```python
from build123d import *

# Parameters (mm, degrees)
F1_DEPTH = 33.02
F2_R     = 5.08
F4_T     = -2.032
F3_R     = 2.794
F5_DEPTH = 2.032


with BuildPart() as f1:
    # F0 (on Top) → F1 (new body)
    with BuildSketch(Plane.XY):
        Polygon((-40.064697, 25.4), (-25.4, 0), (-25.4, 25.4), align=None)
        Polygon((-40.064697, 25.4), (-25.4, 25.4), (-25.4, 50.8), align=None)
        Polygon((-25.4, 0), (0, 0), (0, 50.8), (-25.4, 50.8), (-25.4, 25.4), align=None)
    extrude(amount=F1_DEPTH)

    # F2
    f2_edges = [f1.edges().sort_by_distance(p)[0] for p in [
        (-40.064697, 25.4, 16.51),
        (-25.4, 50.8, 16.51),
        (-25.4, 0, 16.51),
    ]]
    fillet(f2_edges, radius=F2_R)

    # F4
    f4_openings = [f1.faces().sort_by_distance(p)[0] for p in [
        (-16.606713, 25.4, 33.02),
    ]]
    offset(amount=F4_T, openings=f4_openings)

    # F3 (on face) → F5 (cut)
    with BuildSketch(Plane(origin=(0, 0, 0), x_dir=(1, 0, 0), z_dir=(0, 0, -1))):
        with Locations((-11.23353, -25.4)):
            Circle(F3_R)
        with Locations((-11.23353, -38.1)):
            Circle(F3_R)
    extrude(amount=-F5_DEPTH, mode=Mode.SUBTRACT)


solid = f1.part
```
Build history of the part. All positions in model axes, mm. A direction names the side the tool comes from. Coordinates: 2 decimals unless noted, no trailing zeros. Order: outer loops, then holes, each group sorted by start corner. A loop starts at its lowest first (then second) coordinate and runs counter-clockwise, first axis right, second up.
Item 1: Tool access for faces 5 (the cylindrical face through (-11.6, 35.33, 1)), 6 (the flat face through (-12, 2.032, 17)): list every direction of +Z, -Z, +X, -X, +Y, -Y with a clear straight run to the whole face (end or side of a thin tool).
Filled in:
face 5: +Z, -Z
face 6: +Z
Item 2: Saw through at C-C on x = -13. List the corners of the cut face in (y, z), then the cut area to 3 significant figures.
Filled in:
outline: (0, 0) - (23.24, 0) - (23.24, 2.03) - (2.03, 2.03) - (2.03, 33.02) - (0, 33.02) - close; (27.56, 0) - (35.94, 0) - (35.94, 2.03) - (27.56, 2.03) - close; (40.26, 0) - (50.8, 0) - (50.8, 33.02) - (48.77, 33.02) - (48.77, 2.03) - (40.26, 2.03) - close
area: 212 mm2
Item 3: Saw through at A-A on y = 24.5. List the corners of the cut face in (x, z), then the cut area to 3 significant figures.
Filled in:
outline: (-39.2, 0) - (-13.88, 0) - (-13.88, 2.03) - (-37.11, 2.03) - (-37.11, 33.02) - (-39.2, 33.02) - close; (-8.59, 0) - (0, 0) - (0, 33.02) - (-2.03, 33.02) - (-2.03, 2.03) - (-8.59, 2.03) - close
area: 197 mm2
Item 4: Saw through at D-D on x = -4. List the corners of the cut face in (y, z), then the cut area to 3 significant figures.
Filled in:
outline: (0, 0) - (50.8, 0) - (50.8, 33.02) - (48.77, 33.02) - (48.77, 2.03) - (2.03, 2.03) - (2.03, 33.02) - (0, 33.02) - close
area: 229 mm2
Item 5: Drill centre lines: L1, parallel to Y at x = -6.5, z = 3; L2, parallel to X at y = 25.4, z = 0.4; L3, parallel to Z at x = -5, y = 9. Where is each one in solid material? Low to high.
Filled in:
L1: y = 0 to 2.03, 48.77 to 50.8
L2: x = -39.28 to -14.03, -8.44 to 0
L3: z = 0 to 2.03
Item 6: Saw through at B-B on z = 3.5. List the corners of the cut face in (x, y), then the cut area to 3 significant figures.
Filled in:
outline: (-38.6, 22.86) - (-26.87, 2.54) arc R5.08 ccw to (-22.47, 0) - (0, 0) - (0, 50.8) - (-22.47, 50.8) arc R5.08 ccw to (-26.87, 48.26) - (-38.6, 27.94) arc R5.08 ccw to start; hole (-36.84, 23.88) - (-25.11, 3.56) arc R3.05 ccw to (-22.47, 2.03) - (-2.03, 2.03) - (-2.03, 48.77) - (-22.47, 48.77) arc R3.05 ccw to (-25.11, 47.24) - (-36.84, 26.92) arc R3.05 ccw to start
area: 308 mm2
Item 7: Mould opens along Y. For faces 1 (the flat face through (-11, 50.8, 16)), 2 (the flat face through (-1, 26, 33.02)), 3 (the cylindrical face through (-25.04, 0.7, 16.74)), 4 (the flat face through (-31.055, 13.858, 17.309)) say: released by +Y, released by -Y, zero draft, split by the parting line, or undercut.
Filled in:
face 1: released by +Y
face 2: zero draft
face 3: released by -Y
face 4: undercut
Item 8: Drop flat-ended pins along their axis: pin 1 Ø17.5 at (x, y) = (-14.5, 32) entering from +Z; pin 2 Ø5 at (y, z) = (43.5, 19.5) entering from -X; pin 3 Ø8 at (x, z) = (-31.5, 21) entering from +Y. Give the stop position or say it passes through.
Filled in:
pin 1: stops at z = 2.03
pin 2: stops at x = -31.06
pin 3: stops at y = 47.16
